```python
from build123d import *

# Parameters (mm, degrees)
SKETCH_8_W          = 73.42135624
SKETCH_8_H          = 25.5
EXTRUDE_3_DEPTH     = 3
SKETCH_9_R          = 1.5
CUT_EXTRUDE_2_DEPTH = 3


with BuildPart() as part:
    # 草图8 → 凸台-拉伸3 (new body)
    with BuildSketch(Plane(origin=(0, 100, 0), x_dir=(1, 0, 0), z_dir=(0, 1, 0))):
        with Locations((-11.084772404, 22.970398927)):
            Rectangle(SKETCH_8_W, SKETCH_8_H)
    extrude(amount=EXTRUDE_3_DEPTH)

    # 草图9 → 切除-拉伸2 (cut)
    with BuildSketch(Plane(origin=(0, 103, 0), x_dir=(1, 0, 0), z_dir=(0, 1, 0))):
        with Locations(Location((-36.795450524, 18.220398927, 0), (0, 0, 270))):
            Circle(SKETCH_9_R)
        with Locations(Location((14.625905716, 18.220398927, 0), (0, 0, 270))):
            Circle(SKETCH_9_R)
        with Locations(Location((-11.084772404, 18.220398927, 0), (0, 0, 270))):
            Circle(SKETCH_9_R)
    extrude(amount=-CUT_EXTRUDE_2_DEPTH, mode=Mode.SUBTRACT)

    # 草图10 → 放样2 section 0
    with BuildSketch(Plane(origin=(0, 100, 0), x_dir=(1, 0, 0), z_dir=(0, 1, 0))):
        with BuildLine():
            Line((-47.795450524, 35.720398927), (-27.795450524, 35.720398927))
            Line((-27.795450524, 35.720398927), (-47.795450524, 15.720398927))
            Line((-47.795450524, 15.720398927), (-47.795450524, 35.720398927))
        make_face()
    # 草图11 → 放样2 section 1
    with BuildSketch(Plane(origin=(0, 0, 0), x_dir=(1, 0, 0), z_dir=(0, 1, 0))):
        with BuildLine():
            Line((-83.150789583, 71.075737986), (-63.150789583, 71.075737986))
            Line((-63.150789583, 71.075737986), (-83.150789583, 51.075737986))
            Line((-83.150789583, 51.075737986), (-83.150789583, 71.075737986))
        make_face()
    loft_2 = loft()

    # 草图12 → 切除-放样1 section 0
    with BuildSketch(Plane(origin=(0, 100, 0), x_dir=(1, 0, 0), z_dir=(0, 1, 0))):
        with BuildLine():
            Line((-31.33098443, 32.184865021), (-44.259916618, 19.255932833))
            Line((-44.259916618, 19.255932833), (-44.259916618, 32.184865021))
            Line((-44.259916618, 32.184865021), (-31.33098443, 32.184865021))
        make_face()
    # 草图13 → 切除-放样1 section 1
    with BuildSketch(Plane(origin=(0, 0, 0), x_dir=(1, 0, 0), z_dir=(0, 1, 0))):
        with BuildLine():
            Line((-66.686323489, 67.54020408), (-79.615255677, 54.611271892))
            Line((-79.615255677, 54.611271892), (-79.615255677, 67.54020408))
            Line((-79.615255677, 67.54020408), (-66.686323489, 67.54020408))
        make_face()
    loft_1 = loft(mode=Mode.SUBTRACT)

    # 镜向3: 放样2 across plane
    add(loft_2.mirror(Plane(origin=(-11.1, 0, 0), x_dir=(0, 0, 1), z_dir=(1, 0, 0))))

    # 镜向4: 切除-放样1 across plane
    add(loft_1.mirror(Plane(origin=(-11.1, 0, 0), x_dir=(0, 0, 1), z_dir=(1, 0, 0))), mode=Mode.SUBTRACT)


solid = part.part
```
CAD build for the part. Positions are in the model's coordinates, mm. A direction names the side the tool comes from. Give positions to 0.01 mm unless a question says otherwise; leave off trailing zeros.
(1) Mould opens along X. For faces 4 (the flat face through (-47.795, 101, -23)), 5 (the flat face through (41.728, 49.3, -35.438)), 6 (the flat face through (-12, 103, -23)) say: released by +X, released by -X, zero draft, split by the parting line, or undercut.
(2) Tool access for faces 1 (the flat face through (-12, 101, -35.72)), 2 (the flat face through (25.264, 49.3, -51.903)), 3 (the flat face through (25.626, 101, -23)): list every direction of +Z, -Z, +X, -X, +Y, -Y with a clear straight run to the whole face (end or side of a thin tool).
(3) Flat gauge pins, fed straight in: pin 1 (2.5 mm diameter, centred on x = -27, y = 102, fed in from -Z); pin 2 (1.5 mm diameter, centred on y = 102, z = -28.5, fed in from +X); pin 3 (4 mm diameter, centred on x = -36.8, z = -18.22, fed in from +Y); pin 4 (3.5 mm diameter, centred on y = 101.5, z = -28, fed in from -X). Where does each tip first touch, or does it go through?
(4) Drill centre lines: L1, parallel to X at y = 35, z = -44.5; L2, parallel to X at y = 22.5, z = -58; L3, parallel to Y at x = -13.5, z = -25. Where is each one in solid material? Low to high.
Results found:
1. face 4: released by -X
1. face 5: undercut
1. face 6: zero draft
2. face 1: -Z, +X, -X, +Y
2. face 2: +Z, -Y
2. face 3: +Z, -Z, +X, +Y
3. pin 1: stops at z = -35.72
3. pin 2: stops at x = 25.63
3. pin 3: stops at y = 103
3. pin 4: stops at x = -47.88
4. L1: x = -70.78 to -67.24, 45.04 to 48.58
4. L2: x = -75.2 to -71.66, 49.46 to 53
4. L3: y = 100 to 103
